Part model, mm, in its own coordinate system. Coordinates: 2 decimals unless noted, no trailing zeros. Loops run counter-clockwise (first coordinate to the right, second up) from the corner with the lowest first, then second, coordinate; pieces in that order, holes last.
```python
from build123d import *

# Parameters (mm, degrees)
SKETCH1_W           = 120
SKETCH1_H           = 160
SKETCH1_W_2         = 48
SKETCH1_H_2         = 10
SKETCH1_R           = 0.5
SKETCH1_R_2         = 1.75
BOSS_EXTRUDE2_DEPTH = 1.6


with BuildPart() as part:
    # Sketch1 → Boss-Extrude2 (new body)
    with BuildSketch(Plane(origin=(0, 0, 0), x_dir=(1, 0, 0), z_dir=(0, 1, 0))):
        with Locations((60, -80)):
            Rectangle(SKETCH1_W, SKETCH1_H)
        with Locations((46, -60)):
            Rectangle(SKETCH1_W_2, SKETCH1_H_2, mode=Mode.SUBTRACT)
        with Locations((98.497526801, -6.06)):
            Circle(SKETCH1_R, mode=Mode.SUBTRACT)
        with Locations((98.497526801, -3.52)):
            Circle(SKETCH1_R, mode=Mode.SUBTRACT)
        with Locations((98.497526801, -0.98)):
            Circle(SKETCH1_R, mode=Mode.SUBTRACT)
        with Locations((83.257526801, -16.22)):
            Circle(SKETCH1_R, mode=Mode.SUBTRACT)
        with Locations((83.257526801, -13.68)):
            Circle(SKETCH1_R, mode=Mode.SUBTRACT)
        with Locations((83.257526801, -11.14)):
            Circle(SKETCH1_R, mode=Mode.SUBTRACT)
        with Locations((83.257526801, -8.6)):
            Circle(SKETCH1_R, mode=Mode.SUBTRACT)
        with Locations((83.257526801, -6.06)):
            Circle(SKETCH1_R, mode=Mode.SUBTRACT)
        with Locations((83.257526801, -3.52)):
            Circle(SKETCH1_R, mode=Mode.SUBTRACT)
        with Locations((83.257526801, -0.98)):
            Circle(SKETCH1_R, mode=Mode.SUBTRACT)
        with Locations((98.497526801, -16.22)):
            Circle(SKETCH1_R, mode=Mode.SUBTRACT)
        with Locations((98.497526801, -13.68)):
            Circle(SKETCH1_R, mode=Mode.SUBTRACT)
        with Locations((98.497526801, -11.14)):
            Circle(SKETCH1_R, mode=Mode.SUBTRACT)
        with Locations((98.497526801, -8.6)):
            Circle(SKETCH1_R, mode=Mode.SUBTRACT)
        with Locations((12, -82)):
            Circle(SKETCH1_R_2, mode=Mode.SUBTRACT)
        with Locations((12, -156)):
            Circle(SKETCH1_R_2, mode=Mode.SUBTRACT)
        with Locations((54, -82)):
            Circle(SKETCH1_R_2, mode=Mode.SUBTRACT)
        with Locations((39, -82)):
            Circle(SKETCH1_R_2, mode=Mode.SUBTRACT)
        with Locations((39, -156)):
            Circle(SKETCH1_R_2, mode=Mode.SUBTRACT)
        with Locations((54, -156)):
            Circle(SKETCH1_R_2, mode=Mode.SUBTRACT)
        with Locations((108, -82)):
            Circle(SKETCH1_R_2, mode=Mode.SUBTRACT)
        with Locations((108, -156)):
            Circle(SKETCH1_R_2, mode=Mode.SUBTRACT)
        with Locations((66, -82)):
            Circle(SKETCH1_R_2, mode=Mode.SUBTRACT)
        with Locations((81, -156)):
            Circle(SKETCH1_R_2, mode=Mode.SUBTRACT)
        with Locations((81, -82)):
            Circle(SKETCH1_R_2, mode=Mode.SUBTRACT)
        with Locations((66, -156)):
            Circle(SKETCH1_R_2, mode=Mode.SUBTRACT)
    extrude(amount=BOSS_EXTRUDE2_DEPTH)


solid = part.part
```
Q1. Saw through at A-A (y = 1.1). Count the separate pieces of the cut face and the enclosed holes in it, plus the area to 3 significant figures.
Q2. Saw through at B-B (z = 156). List the corners of the cut face in (x, y), plus the area to 3 significant figures.
Q3. Saw through at C-C (x = 26.5). List the corners of the cut face in (y, z), plus the area to 3 significant figures.
Q4. Mould opens along Z. For faces 1 (the flat face through (59, 0, 79)), 2 (the cylindrical face through (55.669, 0.789, 155.474)) say: released by +Z, released by -Z, zero draft, split by the parting line, or undercut.
Q5. Probe line 1 (X direction, y = 0.5, z = 6.06); line 2 (Z direction, x = 54, y = 1.3); line 3 (Z direction, x = 80.5, y = 1.35). List the from-to ranges inside material, lowest first.
Q6. Drop a flat-ended pin along its axis: P1, Ø12, axis at x = 100, z = 128.5, coming from the -Y side. Give the stop position or say it passes through.
Checked values:
1. separate pieces: 1
1. enclosed holes: 27
1. area: 18,600 mm2
2. outline: (0, 0) - (10.25, 0) - (10.25, 1.6) - (0, 1.6) - close; (13.75, 0) - (37.25, 0) - (37.25, 1.6) - (13.75, 1.6) - close; (40.75, 0) - (52.25, 0) - (52.25, 1.6) - (40.75, 1.6) - close; (55.75, 0) - (64.25, 0) - (64.25, 1.6) - (55.75, 1.6) - close; (67.75, 0) - (79.25, 0) - (79.25, 1.6) - (67.75, 1.6) - close; (82.75, 0) - (106.25, 0) - (106.25, 1.6) - (82.75, 1.6) - close; (109.75, 0) - (120, 0) - (120, 1.6) - (109.75, 1.6) - close
2. area: 158 mm2
3. outline: (0, 0) - (1.6, 0) - (1.6, 55) - (0, 55) - close; (0, 65) - (1.6, 65) - (1.6, 160) - (0, 160) - close
3. area: 240 mm2
4. face 1: zero draft
4. face 2: undercut
5. line 1: x = 0 to 82.76, 83.76 to 98, 99 to 120
5. line 2: z = 0 to 55, 65 to 80.25, 83.75 to 154.25, 157.75 to 160
5. line 3: z = 0 to 80.32, 83.68 to 154.32, 157.68 to 160
6. P1: stops at y = 0
